Could you check a few things on this model? Use its own coordinates, in mm. A direction names the side the tool comes from. Give positions to 0.01 mm unless a question says otherwise; leave off trailing zeros. Order: outer loops, then holes, each group sorted by start corner. A loop starts at its lowest first (then second) coordinate and runs counter-clockwise, first axis right, second up. Notation, with made-up numbers: (59.25, 63) -> (98.25, 63) arc R31 cw to (98.25, 98) -> close; hole circle Ø2 at (16.25, 89). An arc over 180 degrees is marked (long way). Use one line per item in the form item = value. Start each with the question number.
from build123d import *

# Parameters (mm, degrees)
BOSS_EXTRUDE1_DEPTH = 5
SKETCH2_R           = 10.25
SKETCH2_R_2         = 1.85
CUT_EXTRUDE1_DEPTH  = 6
SKETCH3_W           = 38
SKETCH3_H           = 5
BOSS_EXTRUDE2_DEPTH = 20
SKETCH4_R           = 3
CUT_EXTRUDE2_DEPTH  = 6


with BuildPart() as part:
    # Sketch1 → Boss-Extrude1 (new body)
    with BuildSketch(Plane.XY):
        with BuildLine():
            Line((-20.15873891, 0), (-20.15873891, -27))
            Line((-20.15873891, -27), (17.84126109, -27))
            Line((17.84126109, -27), (17.84126109, 0))
            ThreePointArc((17.84126109, 0), (-1.15873891, 19), (-20.15873891, 0))
        make_face()
    extrude(amount=BOSS_EXTRUDE1_DEPTH)

    # Sketch2 → Cut-Extrude1 (cut, through all)
    with BuildSketch(Plane(origin=(0, 0, 0), x_dir=(-1, 0, 0), z_dir=(0, 0, -1))):
        with Locations((1.15873891, 0)):
            Circle(SKETCH2_R)
        with Locations((1.15873891, -15.15)):
            Circle(SKETCH2_R_2)
        with Locations((-11.961545957, 7.575)):
            Circle(SKETCH2_R_2)
        with Locations((14.279023778, 7.575)):
            Circle(SKETCH2_R_2)
    extrude(amount=-CUT_EXTRUDE1_DEPTH, mode=Mode.SUBTRACT)

    # Sketch3 → Boss-Extrude2 (add)
    with BuildSketch(Plane(origin=(0, 0, 0), x_dir=(-1, 0, 0), z_dir=(0, 0, -1))):
        with Locations((1.15873891, -24.5)):
            Rectangle(SKETCH3_W, SKETCH3_H)
    extrude(amount=BOSS_EXTRUDE2_DEPTH)

    # Sketch4 → Cut-Extrude2 (cut, through all)
    with BuildSketch(Plane(origin=(0, -22, 0), x_dir=(1, 0, 0), z_dir=(0, 1, 0))):
        with Locations((10.34126109, 10)):
            Circle(SKETCH4_R)
        with Locations((-12.65873891, 10)):
            Circle(SKETCH4_R)
    extrude(amount=-CUT_EXTRUDE2_DEPTH, mode=Mode.SUBTRACT)


solid = part.part
(1) Please list where these lines run through material, in increasing order: probe 1 along X at (y, z) = (-24.3, -10); probe 2 along X at (y, z) = (6, 0.25); probe 3 along Y at (x, z) = (4.5, -3.25).
(2) Imagine slicing it at A-A (z = -10). Write out the boundary of the cut face in (x, y).
(3) We'd pull the mould along X, two halves only. Please class faces 1 (the cylindrical face through (12.2, 9.41, 2.46)), 2 (the flat face through (-20.159, -20, 1)), 3 (the flat face through (-6, -10, 0)): pulls with the +X half, pulls with the -X half, needs draft (parallel to the pull), parting line crosses it, or undercut.
(4) Which directions (+Z, -Z, +X, -X, +Y, -Y) give clear straight access to the entire face, cutting with the end or side of a thin tool? Please do faces 4 (the cylindrical face through (-15.039, -24.465, -8.175)), 5 (the flat face through (-1, -22, -10)).
(5) Imagine slicing it at B-B (y = -15.15). Write out the boundary of the cut face in (x, z), plus the area to 4 significant figures.
(6) Imagine slicing it at D-D (x = -2). Write out the boundary of the cut face in (y, z), plus the area to 3 significant figures.
(7) I'm going to push flat-ended pins straight in: pin 1 Ø5 at (x, z) = (7.5, -13.5) entering from +Y; pin 2 Ø19 at (x, y) = (4.5, -2) entering from -Z. Where does each tip first touch, or does it pass through?
(8) Imagine slicing it at C-C (x = -14.5). Write out the boundary of the cut face in (y, z).
Calculated:
q1.probe_1 = -20.16 to -15.66, -9.66 to 7.34, 13.34 to 17.84
q1.probe_2 = -19.19 to -15.25, -13.31 to -9.47, 7.15 to 10.99, 12.93 to 16.87
q1.probe_3 = -27 to -22
q2.outline = (-20.16, -27) -> (-15.66, -27) -> (-15.66, -22) -> (-20.16, -22) -> close; (-9.66, -27) -> (7.34, -27) -> (7.34, -22) -> (-9.66, -22) -> close; (13.34, -27) -> (17.84, -27) -> (17.84, -22) -> (13.34, -22) -> close
q3.face_1 = undercut
q3.face_2 = pulls with the -X half
q3.face_3 = needs draft
q4.face_4 = +Y, -Y
q4.face_5 = -Z, +X, -X, +Y
q5.outline = (-20.16, 0) -> (-3.01, 0) -> (-3.01, 5) -> (-20.16, 5) -> close; (0.69, 0) -> (17.84, 0) -> (17.84, 5) -> (0.69, 5) -> close
q5.area = 171.5 mm2
q6.outline = (-27, -20) -> (-22, -20) -> (-22, 0) -> (-16.8, 0) -> (-16.8, 5) -> (-27, 5) -> close; (-13.5, 0) -> (-10.22, 0) -> (-10.22, 5) -> (-13.5, 5) -> close; (10.22, 0) -> (18.98, 0) -> (18.98, 5) -> (10.22, 5) -> close
q6.area = 211 mm2
q7.pin_1 = -22
q7.pin_2 = 0
q8.outline = (-27, -20) -> (-22, -20) -> (-22, -12.37) -> (-27, -12.37) -> close; (-27, -7.63) -> (-22, -7.63) -> (-22, 0) -> (5.74, 0) -> (5.74, 5) -> (-27, 5) -> close; (9.41, 0) -> (13.53, 0) -> (13.53, 5) -> (9.41, 5) -> close
